```python
from build123d import *
from OCP.BRepFilletAPI import BRepFilletAPI_MakeChamfer

# Parameters (mm, degrees)
BOSS_EXTRUDE1_DEPTH        = 60
FILLET1_R                  = 2
CHAMFER1_SIZE              = 2
SKETCH2_W                  = 90
SKETCH2_H                  = 30
CUT_EXTRUDE1_DEPTH         = 17.5
CHAMFER2_SIZE              = 15
CHAMFER2_SIZE_2            = 5.459553514
CHAMFER2_OF_MIRROR2_SIZE   = 15
CHAMFER2_OF_MIRROR2_SIZE_2 = 5.459553514


with BuildPart() as part:
    # Sketch1 → Boss-Extrude1 (new body)
    with BuildSketch(Plane.XY):
        with BuildLine():
            Line((0, -76.2), (0, -127))
            Line((0, -127), (60, -127))
            Line((60, -127), (60, -46.972758063))
            ThreePointArc((60, -46.972758063), (33.37001525, -68.504613583), (0, -76.2))
        make_face()
    boss_extrude1 = extrude(amount=BOSS_EXTRUDE1_DEPTH)

    # Mirror1: Boss-Extrude1 across plane
    add(boss_extrude1.mirror(Plane(origin=(0, -76.2, 60), x_dir=(0, 0, 1), z_dir=(1, 0, 0))))

    # Fillet1
    fillet1_edges = [part.edges().sort_by_distance(p)[0] for p in [
        (-60, -46.972758063, 30),
        (60, -46.972758063, 30),
    ]]
    fillet(fillet1_edges, radius=FILLET1_R)

    # Chamfer1
    chamfer1_edges = [part.edges().sort_by_distance(p)[0] for p in [
        (-60, -127, 30),
        (-60, -89.726132006, 60),
        (-60, -89.726132006, 0),
        (0, -76.2, 0),
        (0, -76.2, 60),
        (-58.718765637, -50.585883569, 0),
        (58.718765637, -50.585883569, 0),
        (-58.718765637, -50.585883569, 60),
        (58.718765637, -50.585883569, 60),
        (0, -127, 60),
        (60, -89.726132006, 0),
        (0, -127, 0),
        (60, -127, 30),
        (60, -89.726132006, 60),
    ]]
    chamfer(chamfer1_edges, length=CHAMFER1_SIZE)

    # Sketch2 → Cut-Extrude1 (cut)
    with BuildSketch(Plane(origin=(0, 0, 0), x_dir=(-1, 0, 0), z_dir=(0, 0, -1))):
        with Locations((0, -102)):
            Rectangle(SKETCH2_W, SKETCH2_H)
    cut_extrude1 = extrude(amount=-CUT_EXTRUDE1_DEPTH, mode=Mode.SUBTRACT)

    # Chamfer2
    chamfer2_edges_1 = [part.edges().sort_by_distance(p)[0] for p in [
        (-45, -87, 8.75),
    ]]
    chamfer2_side_1 = [part.faces().sort_by_distance(p)[0] for p in [
        (-44.89080893, -87, 8.75),
    ]]
    chamfer2_edges_2 = [part.edges().sort_by_distance(p)[0] for p in [
        (0, -87, 17.5),
    ]]
    chamfer2_side_2 = [part.faces().sort_by_distance(p)[0] for p in [
        (0, -87, 17.39080893),
    ]]
    chamfer2_edges_3 = [part.edges().sort_by_distance(p)[0] for p in [
        (45, -87, 8.75),
    ]]
    chamfer2_side_3 = [part.faces().sort_by_distance(p)[0] for p in [
        (45, -87.10919107, 8.75),
    ]]
    chamfer2 = BRepFilletAPI_MakeChamfer(part.part.solid().wrapped)
    for e in chamfer2_edges_1:
        chamfer2.Add(CHAMFER2_SIZE - 0.0001, CHAMFER2_SIZE_2 - 0.0001, e.wrapped, chamfer2_side_1[0].wrapped)
    for e in chamfer2_edges_2:
        chamfer2.Add(CHAMFER2_SIZE - 0.0001, CHAMFER2_SIZE_2 - 0.0001, e.wrapped, chamfer2_side_2[0].wrapped)
    for e in chamfer2_edges_3:
        chamfer2.Add(CHAMFER2_SIZE_2 - 0.0001, CHAMFER2_SIZE - 0.0001, e.wrapped, chamfer2_side_3[0].wrapped)
    add(Compound.cast(chamfer2.Shape()), mode=Mode.REPLACE)  # a hair under: the kernel refuses the full size

    # Mirror2: Cut-Extrude1 across plane
    add(cut_extrude1.mirror(Plane(origin=(0, 0, 30), x_dir=(1, 0, 0), z_dir=(0, 0, -1))), mode=Mode.SUBTRACT)

    # Chamfer2 of Mirror2
    chamfer2_of_mirror2_edges_1 = [part.edges().sort_by_distance(p)[0] for p in [
        (-45, -87, 51.25),
    ]]
    chamfer2_of_mirror2_side_1 = [part.faces().sort_by_distance(p)[0] for p in [
        (-44.89080893, -87, 51.25),
    ]]
    chamfer2_of_mirror2_edges_2 = [part.edges().sort_by_distance(p)[0] for p in [
        (0, -87, 42.5),
    ]]
    chamfer2_of_mirror2_side_2 = [part.faces().sort_by_distance(p)[0] for p in [
        (0, -87, 42.60919107),
    ]]
    chamfer2_of_mirror2_edges_3 = [part.edges().sort_by_distance(p)[0] for p in [
        (45, -87, 51.25),
    ]]
    chamfer2_of_mirror2_side_3 = [part.faces().sort_by_distance(p)[0] for p in [
        (45, -87.10919107, 51.25),
    ]]
    chamfer2_of_mirror2 = BRepFilletAPI_MakeChamfer(part.part.solid().wrapped)
    for e in chamfer2_of_mirror2_edges_1:
        chamfer2_of_mirror2.Add(CHAMFER2_OF_MIRROR2_SIZE - 0.0001, CHAMFER2_OF_MIRROR2_SIZE_2 - 0.0001, e.wrapped, chamfer2_of_mirror2_side_1[0].wrapped)
    for e in chamfer2_of_mirror2_edges_2:
        chamfer2_of_mirror2.Add(CHAMFER2_OF_MIRROR2_SIZE - 0.0001, CHAMFER2_OF_MIRROR2_SIZE_2 - 0.0001, e.wrapped, chamfer2_of_mirror2_side_2[0].wrapped)
    for e in chamfer2_of_mirror2_edges_3:
        chamfer2_of_mirror2.Add(CHAMFER2_OF_MIRROR2_SIZE_2 - 0.0001, CHAMFER2_OF_MIRROR2_SIZE - 0.0001, e.wrapped, chamfer2_of_mirror2_side_3[0].wrapped)
    add(Compound.cast(chamfer2_of_mirror2.Shape()), mode=Mode.REPLACE)  # a hair under: the kernel refuses the full size


solid = part.part
```
Work out the finished part from the listing and answer in its coordinate system (mm). A direction names the side the tool comes from. Give positions to 0.01 mm unless a question says otherwise; leave off trailing zeros. Loops run counter-clockwise (first coordinate to the right, second up) from the corner with the lowest first, then second, coordinate; pieces in that order, holes last. Notation, with made-up numbers: M 54,-18.75 L 82,-18.75 A15 cw 82,6.25 Z; hole C -29,-1.5 d3. An arc over 180 degrees is marked long. One line per item, written item: value. Start each with the question number.
1. Find section A-A (y = -98.5). Give the vertices of the cut face in (x, z), and give its area (3 significant figures).
2. Each of these flat-tipped pins is pushed along its axis until it touches: P1, Ø12.5, axis at x = -14.5, y = -101.5, coming from the +Z side; P2, Ø5, axis at x = 3.5, z = 48.5, coming from the +Y side; P3, Ø19, axis at x = 1, z = 7.5, coming from the +Y side. Where does it stop, or does it pass through?
3. Find section C-C (z = 48.5). Give the vertices of the cut face in (x, y).
4. Find section B-B (z = 29.5). Give the vertices of the cut face in (x, y).
5. Determine the mould class of faces 4 (the face through (-60, -89, 30)), 5 (the face through (1, -80, 60)), 6 (the face through (-45, -105, 9)) for opening direction X: released by +X, released by -X, zero draft, split by the parting line, or undercut.
6. Find the intervals of material crossed by probe 1 along X at (y, z) = (-102, 50.5); probe 2 along Y at (x, z) = (-20.5, 14); probe 3 along X at (y, z) = (-60, 39), in increasing order.
7. Which of the six approach directions +Z, -Z, +X, -X, +Y, -Y give full straight-line access (tool end or side, diameter ignored) to faces 1 (the face through (39.062, -90.298, 6.683)), 2 (the face through (39.062, -90.298, 53.317)), 3 (the face through (1, -127, 30))?
Reported:
1. outline: M -60,2 L -58,0 L -45,0 L -45,17.5 L 45,17.5 L 45,0 L 58,0 L 60,2 L 60,58 L 58,60 L 45,60 L 45,42.5 L -45,42.5 L -45,60 L -58,60 L -60,58 Z
1. area: 4,040 mm²
2. P1: stops at z = 42.5
2. P2: stops at y = -75.96
2. P3: stops at y = -75.47
3. outline: M -60,-125 L -58,-127 L 58,-127 L 60,-125 L 60,-52.45 A2 ccw 56.52,-51.11 A76.2 cw -56.52,-51.11 A2 ccw -60,-52.45 Z; hole M -45,-117 L 45,-117 L 45,-92.46 L 39,-90.28 L -39,-90.28 L -45,-92.46 Z
4. outline: M -60,-125 L -58,-127 L 58,-127 L 60,-125 L 60,-52.45 A2 ccw 56.52,-51.11 A76.2 cw -56.52,-51.11 A2 ccw -60,-52.45 Z
5. face 4: released by -X
5. face 5: zero draft
5. face 6: undercut
6. probe 1: x = -60 to -45, 45 to 60
6. probe 2: y = -127 to -117, -91.19 to -73.39
6. probe 3: x = -60 to -46.97, 46.97 to 60
7. face 1: -Z
7. face 2: +Z
7. face 3: +Z, -Z, +X, -X, -Y
